Source: CAD feature listing. Evaluate the final solid. Frame: model axes, mm. A direction names the side the tool comes from. Give positions to 0.01 mm unless a question says otherwise; leave off trailing zeros. Loops run counter-clockwise (first coordinate to the right, second up) from the corner with the lowest first, then second, coordinate; pieces in that order, holes last. Notation, with made-up numbers: M 87,4.25 L 132,4.25 A23 cw 132,23.25 Z; hole C 83,-32 d6. An arc over 180 degrees is marked long. Put each result on its own line as item: value. Start each with the question number.
```python
from build123d import *

# Parameters (mm, degrees)
CYLINDER1675_R              = 1.5
CYLINDER1675_DEPTH          = 20
CYLINDER1676_R              = 1.5
CYLINDER1676_DEPTH          = 20
COMPOUND830_ROLL_ANGLE      = 90
COMPOUND830_PLACEMENT_ANGLE = 90
CYLINDER1665_R              = 2.5
CYLINDER1665_DEPTH          = 20
CYLINDER1664_R              = 2.5
CYLINDER1664_DEPTH          = 20
CYLINDER1663_R              = 5
CYLINDER1663_DEPTH          = 5
CYLINDER1662_R              = 5
CYLINDER1662_DEPTH          = 5
CYLINDER1659_R              = 3
CYLINDER1659_DEPTH          = 3
CYLINDER1660_R              = 3
CYLINDER1660_DEPTH          = 3
CYLINDER1661_R              = 3
CYLINDER1661_DEPTH          = 3
CYLINDER1658_R              = 3
CYLINDER1658_DEPTH          = 3
CYLINDER1651_R              = 1.5
CYLINDER1651_DEPTH          = 60
CYLINDER1652_R              = 1.5
CYLINDER1652_DEPTH          = 60
CYLINDER1653_R              = 1.5
CYLINDER1653_DEPTH          = 60
CYLINDER1650_R              = 1.5
CYLINDER1650_DEPTH          = 60
CYLINDER1617_R              = 5
CYLINDER1617_DEPTH          = 5
BOX643_W                    = 90
BOX643_H                    = 20
BOX643_DEPTH                = 4
CHAMFER040_SIZE             = 4
CHAMFER041_SIZE             = 2


with BuildPart() as obj1:
    # Cylinder1675 → Cylinder1675 (new body)
    with BuildSketch(Plane(origin=(15.75, 114, 58.525), x_dir=(-1, 0, 0), z_dir=(0, 1, 0))):
        Circle(CYLINDER1675_R)
    extrude(amount=CYLINDER1675_DEPTH)


with BuildPart() as compound831:
    # Cylinder1676 → Cylinder1676 (new body)
    with BuildSketch(Plane(origin=(15.75, 114, 39.475), x_dir=(-1, 0, 0), z_dir=(0, 1, 0))):
        Circle(CYLINDER1676_R)
    extrude(amount=CYLINDER1676_DEPTH)

    # Compound830: union obj1
    add(obj1.part)


with BuildPart() as compound831_1:
    # Compound830 roll: moved
    add(compound831.part.rotate(Axis((0, 0, 0), (1, 0, 0)), COMPOUND830_ROLL_ANGLE))


with BuildPart() as compound831_2:
    # Compound830 placement: moved
    add(compound831_1.part.moved(Location((-49, 0, -96))).rotate(Axis((-49, 0, -96), (0, 0, 1)), COMPOUND830_PLACEMENT_ANGLE))


with BuildPart() as compound831_3:
    # Compound831 placement: moved
    add(compound831_2.part.moved(Location((0, 74, -72))))


with BuildPart() as obj2:
    # Cylinder1665 → Cylinder1665 (new body)
    with BuildSketch(Plane(origin=(-35, 90, -59), x_dir=(1, 0, 0), z_dir=(0, 0, 1))):
        Circle(CYLINDER1665_R)
    extrude(amount=CYLINDER1665_DEPTH)


with BuildPart() as compound817:
    # Cylinder1664 → Cylinder1664 (new body)
    with BuildSketch(Plane(origin=(35, 90, -59), x_dir=(1, 0, 0), z_dir=(0, 0, 1))):
        Circle(CYLINDER1664_R)
    extrude(amount=CYLINDER1664_DEPTH)

    # Compound817: union obj2
    add(obj2.part)


with BuildPart() as obj3:
    # Cylinder1663 → Cylinder1663 (new body)
    with BuildSketch(Plane(origin=(-35, 90, -59), x_dir=(1, 0, 0), z_dir=(0, 0, 1))):
        Circle(CYLINDER1663_R)
    extrude(amount=CYLINDER1663_DEPTH)


with BuildPart() as compound816:
    # Cylinder1662 → Cylinder1662 (new body)
    with BuildSketch(Plane(origin=(35, 90, -59), x_dir=(1, 0, 0), z_dir=(0, 0, 1))):
        Circle(CYLINDER1662_R)
    extrude(amount=CYLINDER1662_DEPTH)

    # Compound816: union obj3
    add(obj3.part)


with BuildPart() as obj4:
    # Cylinder1659 → Cylinder1659 (new body)
    with BuildSketch(Plane(origin=(18, 85, -57), x_dir=(1, 0, 0), z_dir=(0, 0, 1))):
        Circle(CYLINDER1659_R)
    extrude(amount=CYLINDER1659_DEPTH)


with BuildPart() as obj5:
    # Cylinder1660 → Cylinder1660 (new body)
    with BuildSketch(Plane(origin=(-18, 85, -57), x_dir=(1, 0, 0), z_dir=(0, 0, 1))):
        Circle(CYLINDER1660_R)
    extrude(amount=CYLINDER1660_DEPTH)


with BuildPart() as obj6:
    # Cylinder1661 → Cylinder1661 (new body)
    with BuildSketch(Plane(origin=(-18, 95, -57), x_dir=(1, 0, 0), z_dir=(0, 0, 1))):
        Circle(CYLINDER1661_R)
    extrude(amount=CYLINDER1661_DEPTH)


with BuildPart() as compound815:
    # Cylinder1658 → Cylinder1658 (new body)
    with BuildSketch(Plane(origin=(18, 95, -57), x_dir=(1, 0, 0), z_dir=(0, 0, 1))):
        Circle(CYLINDER1658_R)
    extrude(amount=CYLINDER1658_DEPTH)

    # Compound815: union obj4, obj5, obj6
    add(obj4.part)
    add(obj5.part)
    add(obj6.part)


with BuildPart() as obj7:
    # Cylinder1651 → Cylinder1651 (new body)
    with BuildSketch(Plane(origin=(18, 85, -57), x_dir=(1, 0, 0), z_dir=(0, 0, 1))):
        Circle(CYLINDER1651_R)
    extrude(amount=CYLINDER1651_DEPTH)


with BuildPart() as obj8:
    # Cylinder1652 → Cylinder1652 (new body)
    with BuildSketch(Plane(origin=(-18, 85, -57), x_dir=(1, 0, 0), z_dir=(0, 0, 1))):
        Circle(CYLINDER1652_R)
    extrude(amount=CYLINDER1652_DEPTH)


with BuildPart() as obj9:
    # Cylinder1653 → Cylinder1653 (new body)
    with BuildSketch(Plane(origin=(-18, 95, -57), x_dir=(1, 0, 0), z_dir=(0, 0, 1))):
        Circle(CYLINDER1653_R)
    extrude(amount=CYLINDER1653_DEPTH)


with BuildPart() as compound813:
    # Cylinder1650 → Cylinder1650 (new body)
    with BuildSketch(Plane(origin=(18, 95, -57), x_dir=(1, 0, 0), z_dir=(0, 0, 1))):
        Circle(CYLINDER1650_R)
    extrude(amount=CYLINDER1650_DEPTH)

    # Compound813: union obj7, obj8, obj9
    add(obj7.part)
    add(obj8.part)
    add(obj9.part)


with BuildPart() as obj10:
    # Cylinder1617 → Cylinder1617 (new body)
    with BuildSketch(Plane(origin=(0, 90, -54), x_dir=(1, 0, 0), z_dir=(0, 0, 1))):
        Circle(CYLINDER1617_R)
    extrude(amount=CYLINDER1617_DEPTH)


with BuildPart() as cut335:
    # Box643 → Box643 (new body)
    with BuildSketch(Plane(origin=(-45, 80, -56), x_dir=(1, 0, 0), z_dir=(0, 0, 1))):
        with Locations((45, 10)):
            Rectangle(BOX643_W, BOX643_H)
    extrude(amount=BOX643_DEPTH)

    # Cut310: cut obj10
    add(obj10.part, mode=Mode.SUBTRACT)

    # Cut326: cut Compound813
    add(compound813.part, mode=Mode.SUBTRACT)

    # Cut328: cut Compound815
    add(compound815.part, mode=Mode.SUBTRACT)

    # Cut329: cut Compound816
    add(compound816.part, mode=Mode.SUBTRACT)

    # Cut330: cut Compound817
    add(compound817.part, mode=Mode.SUBTRACT)

    # Chamfer040
    chamfer040_edges = [cut335.edges().sort_by_distance(p)[0] for p in [
        (-45, 100, -54),
        (45, 100, -54),
    ]]
    chamfer(chamfer040_edges, length=CHAMFER040_SIZE)

    # Chamfer041
    chamfer041_edges = [cut335.edges().sort_by_distance(p)[0] for p in [
        (-45, 88, -56),
        (45, 88, -56),
    ]]
    chamfer(chamfer041_edges, length=CHAMFER041_SIZE)

    # Cut335: cut Compound831
    add(compound831_3.part, mode=Mode.SUBTRACT)


solid = cut335.part
```
1. Ray query, line 1 (Y direction, x = -18, z = -53.4); line 2 (Y direction, x = 18, z = -54.85); line 3 (X direction, y = 89.75, z = -53.2) (3 decimals). Return the intervals inside material, ascending.
2. Pull-direction query (Y, two-part tool) for faces 1 (the face through (-1, 90, -56)), 2 (the face through (34.67, 92.48, -53.01)), 3 (the face through (-1, 80, -54)); classes: released by +Y, released by -Y, zero draft, split by the parting line, or undercut.
3. Section C-C, the plane z = -55.05. Output: boundary loops of the cut face in (x, y).
4. Section D-D, the plane x = 0. Output: boundary loops of the cut face in (y, z), plus the area to 3 significant figures.
5. Set-up query: faces 4 (the face through (-18.195, 96.487, -53.014)), 5 (the face through (0, 90, -54)), 6 (the face through (31, 87, -55)). Return all of +Z, -Z, +X, -X, +Y, -Y with unobstructed straight access to the full face (end or side cutting, diameter ignored); none if empty.
6. Contact query for flat-ended pins moving along their axis: pin 1 (4 mm diameter, centred on x = 35, y = 90, fed in from -Z); pin 2 (1.8 mm diameter, centred on x = 9.525, y = 89.75, fed in from +Z). Output: stop coordinate, or through.
7. Section A-A, the plane x = -35. Output: boundary loops of the cut face in (y, z), plus the area to 3 significant figures.
8. Section B-B, the plane x = -18. Output: boundary loops of the cut face in (y, z).
Results found:
1. line 1: 80 to 83.5, 86.5 to 93.5, 96.5 to 100
1. line 2: 80 to 82, 88 to 92, 98 to 100
1. line 3: -45 to -37.487, -32.513 to -11.025, -8.025 to -4.994, 4.994 to 8.025, 11.025 to 32.513, 37.487 to 45
2. face 1: zero draft
2. face 2: undercut
2. face 3: released by -Y
3. outline: M -43.95,80 L 43.95,80 L 43.95,97.05 L 41,100 L -41,100 L -43.95,97.05 Z; hole C -35,90 d10; hole C -18,85 d6; hole C -18,95 d6; hole C 18,85 d6; hole C 18,95 d6; hole C 35,90 d10
4. outline: M 80,-56 L 100,-56 L 100,-52 L 95,-52 L 95,-54 L 85,-54 L 85,-52 L 80,-52 Z
4. area: 60.0 mm²
5. face 4: +Z, -Z
5. face 5: +Z
5. face 6: -Z
6. pin 1: through
6. pin 2: z = -54
7. outline: M 80,-56 L 85,-56 L 85,-54 L 87.5,-54 L 87.5,-52 L 80,-52 Z; M 92.5,-54 L 95,-54 L 95,-56 L 100,-56 L 100,-52 L 92.5,-52 Z
7. area: 50.0 mm²
8. outline: M 80,-56 L 82,-56 L 82,-54 L 83.5,-54 L 83.5,-52 L 80,-52 Z; M 86.5,-54 L 88,-54 L 88,-56 L 92,-56 L 92,-54 L 93.5,-54 L 93.5,-52 L 86.5,-52 Z; M 96.5,-54 L 98,-54 L 98,-56 L 100,-56 L 100,-52 L 96.5,-52 Z
